Check sheet for the modelled part. Datum: model origin and axes. Units: mm. A direction names the side the tool comes from. Coordinates: 2 decimals unless noted, no trailing zeros. Order: outer loops, then holes, each group sorted by start corner. A loop starts at its lowest first (then second) coordinate and runs counter-clockwise, first axis right, second up. Notation, with made-up numbers: (65.25, 35.25) -> (101.25, 35.25) arc R8 cw to (101.25, 46.25) -> close; hole circle Ø7 at (62, 18). An arc over 180 degrees is marked (long way). Put each result on its own line as item: value. Start each with the question number.
```python
from build123d import *

# Parameters (mm, degrees)
SKETCH_R     = 2.5
PAD_DEPTH    = 2
FILLET_R     = 1
SKETCH001_R  = 1.5
PAD001_DEPTH = 10
SKETCH002_R  = 0.75
POCKET_DEPTH = 3


with BuildPart() as part:
    # Sketch → Pad (new body)
    with BuildSketch(Plane.XY):
        Circle(SKETCH_R)
    extrude(amount=PAD_DEPTH)

    # Fillet
    fillet_edges = [part.edges().sort_by_distance(p)[0] for p in [
        (-2.5, 0, 0),
    ]]
    fillet(fillet_edges, radius=FILLET_R)

    # Sketch001 (on DatumPlane) → Pad001 (join)
    with BuildSketch(Plane.XY.offset(2)):
        Circle(SKETCH001_R)
    extrude(amount=PAD001_DEPTH)

    # Sketch002 (on DatumPlane) → Pocket (cut)
    with BuildSketch(Plane.XY.offset(12)):
        Circle(SKETCH002_R)
    extrude(amount=-POCKET_DEPTH, mode=Mode.SUBTRACT)


solid = part.part
```
1) Gauge pin test, flat end, axial feed: pin 1 (2 mm diameter, centred on x = -2, z = 3.5, fed in from +Y). Record the tip position at first contact, or that the pin passes through.
2) Access from +Z, -Z, +X, -X, +Y, -Y to the whole of each face (thin tool, end or side, straight path). Record for faces 1 (the flat face through (0, 0, 0)), 2 (the cylindrical face through (-1.5, 0.07, 6.93)).
3) Mould release check, pull along X, two halves, no side actions. Record for faces 3 (the flat face through (-1, 0, 12)), 4 (the cylindrical face through (-0.75, 0.03, 10.52)), 5 (the cylindrical face through (-0.54, -2.44, 1.49)), 6 (the flat face through (0, 0, 9)): +X half, -X half, draft (parallel to the pull), parting line (faces both ways), or undercut.
4) Sectioned sample at D-D (z = 3). Record the boundary of the cut face in (x, y), plus the area to 3 significant figures.
5) Sectioned sample at A-A (y = 0). Record the boundary of the cut face in (x, z), plus the area to 3 significant figures.
6) Sectioned sample at C-C (z = 9.75). Record the boundary of the cut face in (x, y), plus the area to 3 significant figures.
7) Scan lines: line 1 along Z through (x, y) = (0.6, 0.4); line 2 along X through (y, z) = (0.6, 11); line 3 along Z through (x, y) = (1.1, -1.6). Record each from-to range of solid material in increasing order. Write a range as [from, to].
Entries:
1. pin 1: stops at y = 1.12
2. face 1: -Z, +X, -X, +Y, -Y
2. face 2: +Z
3. face 3: draft
3. face 4: undercut
3. face 5: parting line
3. face 6: undercut
4. outline: circle Ø3 at (0, 0)
4. area: 7.07 mm2
5. outline: (-2.5, 1) arc R1 ccw to (-1.5, 0) -> (1.5, 0) arc R1 ccw to (2.5, 1) -> (2.5, 2) -> (1.5, 2) -> (1.5, 12) -> (0.75, 12) -> (0.75, 9) -> (-0.75, 9) -> (-0.75, 12) -> (-1.5, 12) -> (-1.5, 2) -> (-2.5, 2) -> close
5. area: 35.1 mm2
6. outline: circle Ø3 at (0, 0); hole circle Ø1.5 at (0, 0)
6. area: 5.30 mm2
7. line 1: z = [0, 9]
7. line 2: x = [-1.37, -0.45], [0.45, 1.37]
7. line 3: z = [0.1, 2]
